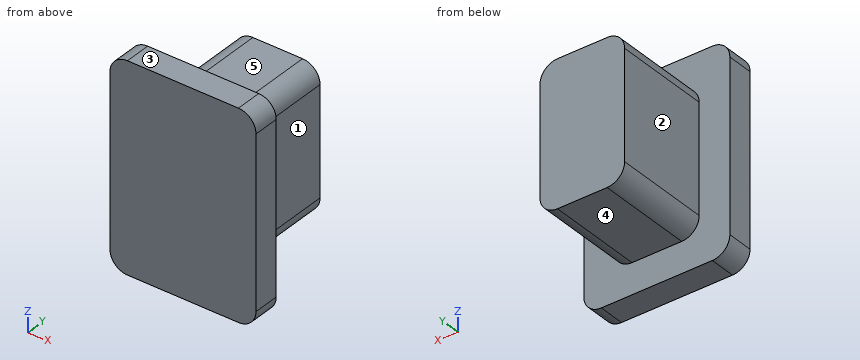
from build123d import *

# Parameters (mm, degrees)
SKETCH_1_W      = 5
SKETCH_1_H      = 7
EXTRUDE_1_DEPTH = 0.9
SKETCH_2_W      = 2.9
SKETCH_2_H      = 4.9
EXTRUDE_2_DEPTH = 3.32
FILLET_1_R      = 0.6


with BuildPart() as part:
    # 草图1 → 凸台-拉伸1 (new body)
    with BuildSketch(Plane(origin=(0, 0, 0), x_dir=(1, 0, 0), z_dir=(0, 1, 0))):
        Rectangle(SKETCH_1_W, SKETCH_1_H)
    extrude(amount=EXTRUDE_1_DEPTH)

    # 草图2 → 凸台-拉伸2 (add)
    with BuildSketch(Plane(origin=(0, 0.9, 0), x_dir=(1, 0, 0), z_dir=(0, 1, 0))):
        Rectangle(SKETCH_2_W, SKETCH_2_H)
    extrude(amount=EXTRUDE_2_DEPTH)

    # 圆角1
    fillet_1_edges = [part.edges().sort_by_distance(p)[0] for p in [
        (1.45, 2.56, 2.45),
        (1.45, 2.56, -2.45),
        (-1.45, 2.56, -2.45),
        (-1.45, 2.56, 2.45),
        (2.5, 0.45, 3.5),
        (-2.5, 0.45, 3.5),
        (-2.5, 0.45, -3.5),
        (2.5, 0.45, -3.5),
    ]]
    fillet(fillet_1_edges, radius=FILLET_1_R)


solid = part.part
The listing builds one solid part. Answer for the finished solid, in the listing's coordinates (mm). Face numbers are marked on the shaded views. A direction names the side the tool comes from. Give positions to 0.01 mm unless a question says otherwise; leave off trailing zeros. Order: outer loops, then holes, each group sorted by start corner. A loop starts at its lowest first (then second) coordinate and runs counter-clockwise, first axis right, second up. Notation, with made-up numbers: (-22.75, 51) -> (9.25, 51) arc R30 ccw to (9.25, 89) -> close; hole circle Ø5 at (-11.75, -1). An arc over 180 degrees is marked (long way). Put each result on its own line as item: value.
Item 1: Given P1, Ø0.8, axis at x = -0.5, y = 3, coming from the +Z side; P2, Ø2.5, axis at y = 2.5, z = 1, coming from the -X side; P3, Ø2.5, axis at y = 2.5, z = -0.5, coming from the +X side, each flat-ended and moving along its own axis, determine where each tip first touches the part or whether it passes through.
Established:
P1: stops at z = 2.45
P2: stops at x = -1.45
P3: stops at x = 1.45
Item 2: A cutting plane is placed at D-D on z = 3.25. Give the vertices of the cut face in (x, y), plus the area to 3 significant figures.
Established:
outline: (-2.39, 0) -> (2.39, 0) -> (2.39, 0.9) -> (-2.39, 0.9) -> close
area: 4.30 mm^2
Item 3: For the marked faces 1, 2, 3, 4 and 5, determine the directions among +Z, -Z, +X, -X, +Y, -Y from which every point of the face is accessible in a straight line to the end or side of a thin tool.
Established:
face 1: +Z, -Z, +X, +Y
face 2: +Z, -Z, -X, +Y
face 3: +Z, +X, -X, +Y, -Y
face 4: -Z, +X, -X, +Y
face 5: +Z, +X, -X, +Y
Item 4: A cutting plane is placed at C-C on x = 1.7. Give the vertices of the cut face in (y, z), plus the area to 3 significant figures.
Established:
outline: (0, -3.5) -> (0.9, -3.5) -> (0.9, 3.5) -> (0, 3.5) -> close
area: 6.30 mm^2
Item 5: A cutting plane is placed at B-B on z = -1.5. Give the vertices of the cut face in (x, y), plus the area to 3 significant figures.
Established:
outline: (-2.5, 0) -> (2.5, 0) -> (2.5, 0.9) -> (1.45, 0.9) -> (1.45, 4.22) -> (-1.45, 4.22) -> (-1.45, 0.9) -> (-2.5, 0.9) -> close
area: 14.1 mm^2
Item 6: Straight lines are drawn through the part: line 1 (X direction, y = 2.9, z = -1.5); line 2 (Y direction, x = 0.15, z = 3.25); line 3 (Z direction, x = 0.6, y = 3.05). For each, find the intervals that lie inside material, in ascending order.
Established:
line 1: x = -1.45 to 1.45
line 2: y = 0 to 0.9
line 3: z = -2.45 to 2.45
Item 7: A cutting plane is placed at A-A on y = 3.1. Give the vertices of the cut face in (x, z), plus the area to 3 significant figures.
Established:
outline: (-1.45, -1.85) arc R0.6 ccw to (-0.85, -2.45) -> (0.85, -2.45) arc R0.6 ccw to (1.45, -1.85) -> (1.45, 1.85) arc R0.6 ccw to (0.85, 2.45) -> (-0.85, 2.45) arc R0.6 ccw to (-1.45, 1.85) -> close
area: 13.9 mm^2
